Work out the finished part from the listing and answer in its coordinate system (mm). Face numbers are marked on the shaded views. Give positions to 0.01 mm unless a question says otherwise; leave off trailing zeros. Loops run counter-clockwise (first coordinate to the right, second up) from the corner with the lowest first, then second, coordinate; pieces in that order, holes last.
```python
from build123d import *

# Parameters (mm, degrees)
F1_DEPTH = 25.4


with BuildPart() as f1:
    # F0 (on Front) → F1 (new body)
    with BuildSketch(Plane.XZ):
        with BuildLine():
            Line((-22.413391, -1.969051), (0, -24.382442))
            Line((0, -24.382442), (22.413391, -1.969051))
            ThreePointArc((22.413391, -1.969051), (24.785195, 1.764316), (25.345929, 6.151691))
            ThreePointArc((25.345929, 6.151691), (12.11404, 17.667495), (0, 4.98102))
            ThreePointArc((0, 4.98102), (-12.11404, 17.667495), (-25.345929, 6.151691))
            ThreePointArc((-25.345929, 6.151691), (-24.785195, 1.764316), (-22.413391, -1.969051))
        make_face()
    extrude(amount=F1_DEPTH)


solid = f1.part
```
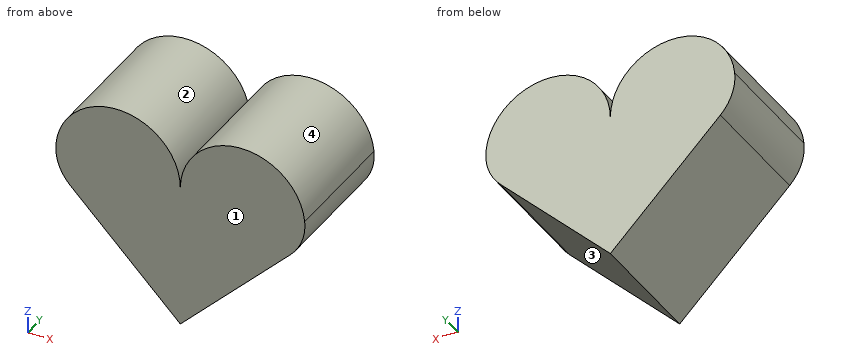
Q1. Determine the mould class of the marked faces 1, 2, 3 and 4 for opening direction X: +X half, -X half, draft (parallel to the pull), parting line (faces both ways), or undercut.
Q2. Section A-A on z = 9 is taken. Give the vertices of the cut face in (x, y), plus the area to 3 significant figures.
Q3. Section D-D on z = -13 is taken. Give the vertices of the cut face in (x, y), plus the area to 3 significant figures.
Q4. Given pin 1 (12 mm diameter, centred on y = -15.5, z = -10, fed in from -X); pin 2 (8 mm diameter, centred on x = -16, z = -4, fed in from +Y); pin 3 (4 mm diameter, centred on y = -22, z = 9.5, fed in from -X); pin 4 (1.5 mm diameter, centred on y = -15, z = -9.5, fed in from -X), each flat-ended and moving along its own axis, determine where each tip first touches the part or whether it passes through.
Q5. Section B-B on y = -5 is taken. Give the vertices of the cut face in (x, z).
Q6. Consider line 1 along X through (y, z) = (-6, 11.5); line 2 along X through (y, z) = (-17.25, 10); line 3 along X through (y, z) = (-3.5, -19). Determine where each line is inside the solid, lowest interval first.
Q7. Section C-C on x = 12.7 is taken. Give the vertices of the cut face in (y, z), plus the area to 3 significant figures.
Check result:
1. face 1: draft
1. face 2: undercut
1. face 3: +X half
1. face 4: undercut
2. outline: (-24.75, -25.4) - (-0.65, -25.4) - (-0.65, 0) - (-24.75, 0) - close; (0.65, -25.4) - (24.75, -25.4) - (24.75, 0) - (0.65, 0) - close
2. area: 1,220 mm2
3. outline: (-11.38, -25.4) - (11.38, -25.4) - (11.38, 0) - (-11.38, 0) - close
3. area: 578 mm2
4. pin 1: stops at x = -20.38
4. pin 2: stops at y = 0
4. pin 3: stops at x = -25.15
4. pin 4: stops at x = -15.63
5. outline: (-25.35, 6.15) arc R10.16 ccw to (-22.41, -1.97) - (0, -24.38) - (22.41, -1.97) arc R10.16 ccw to (25.35, 6.15) arc R12.7 ccw to (0, 4.98) arc R12.7 ccw to start
6. line 1: x = -23.6 to -1.8, 1.8 to 23.6
6. line 2: x = -24.37 to -1.03, 1.03 to 24.37
6. line 3: x = -5.38 to 5.38
7. outline: (-25.4, -11.68) - (0, -11.68) - (0, 17.68) - (-25.4, 17.68) - close
7. area: 746 mm2
